Geometry: final body of the model. Coordinates: model frame, mm. Face numbers are marked on the shaded views. A direction names the side the tool comes from. Give positions to 0.01 mm unless a question says otherwise; leave off trailing zeros. Write each loop counter-clockwise with the first axis right and the second up, starting at its lowest first coordinate (ties: lowest second). Pieces come first, ordered by that corner, then holes.
from build123d import *

# Parameters (mm, degrees)
SKETCH5_R          = 25
CUT_EXTRUDE2_DEPTH = 100
SKETCH6_W          = 54.11225924
SKETCH6_H          = 36.891131312
CUT_EXTRUDE3_DEPTH = 75


with BuildPart() as part:
    # Sketch4 → Revolve2 (revolve)
    with BuildSketch(Plane.XY, mode=Mode.PRIVATE) as revolve2_sk:
        Polygon((0, -251.612903226), (0, -151.612903226), (100, -151.612903226), (100, 48.387096774), (152.822580645, 48.387096774), (200, 48.387096774), (200, -1.612903226), (150, -1.612903226), (150, -151.612903226), (300, -151.612903226), (300, -251.612903226), align=None)
    revolve(revolve2_sk.sketch.rotate(Axis((0, -251.612903226, 0), (0, 1, 0)), 90), axis=Axis((0, -251.612903226, 0), (0, 1, 0)))

    # Sketch5 → Cut-Extrude2 (cut)
    with BuildSketch(Plane(origin=(0, -151.612903226, 0), x_dir=(1, 0, 0), z_dir=(0, 1, 0))):
        with Locations(Location((0, 255.365455535, 0), (0, 0, 270))):
            Circle(SKETCH5_R)
        with Locations(Location((255.365455535, 0, 0), (0, 0, 270))):
            Circle(SKETCH5_R)
        with Locations(Location((0, -255.365455535, 0), (0, 0, 270))):
            Circle(SKETCH5_R)
        with Locations(Location((-255.365455535, 0, 0), (0, 0, 270))):
            Circle(SKETCH5_R)
    extrude(amount=-CUT_EXTRUDE2_DEPTH, mode=Mode.SUBTRACT)

    # Sketch6 → Cut-Extrude3 (cut)
    with BuildSketch(Plane(origin=(0, 48.387096774, 0), x_dir=(1, 0, 0), z_dir=(0, 1, 0))):
        with Locations((200, 0)):
            Rectangle(SKETCH6_W, SKETCH6_H)
    extrude(amount=-CUT_EXTRUDE3_DEPTH, mode=Mode.SUBTRACT)


solid = part.part
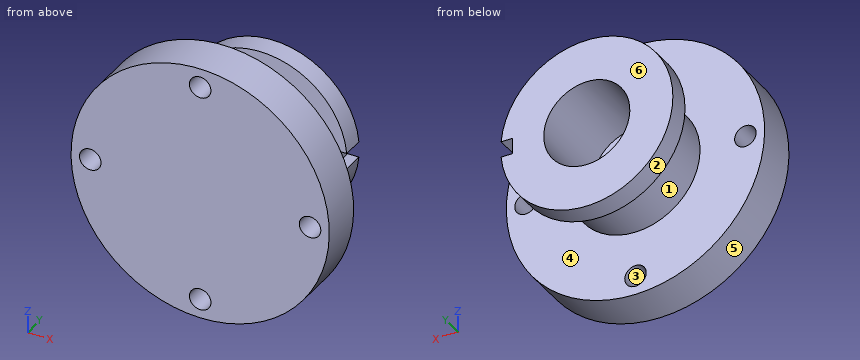
Q1. Section D-D on x = 263. Output: boundary loops of the cut face in (y, z).
Filled sheet:
outline: (-251.61, -144.33) - (-151.61, -144.33) - (-151.61, -23.81) - (-251.61, -23.81) - close; (-251.61, 23.81) - (-151.61, 23.81) - (-151.61, 144.33) - (-251.61, 144.33) - close
Q2. Section A-A on z = 0. Output: boundary loops of the cut face in (x, y), plus the area to 3 significant figures.
Filled sheet:
outline: (-300, -251.61) - (-280.37, -251.61) - (-280.37, -151.61) - (-300, -151.61) - close; (-230.37, -251.61) - (230.37, -251.61) - (230.37, -151.61) - (150, -151.61) - (150, -1.61) - (172.94, -1.61) - (172.94, 48.39) - (100, 48.39) - (100, -151.61) - (-100, -151.61) - (-100, 48.39) - (-200, 48.39) - (-200, -1.61) - (-150, -1.61) - (-150, -151.61) - (-230.37, -151.61) - close; (280.37, -251.61) - (300, -251.61) - (300, -151.61) - (280.37, -151.61) - close
area: 73,600 mm2
Q3. Ray query, line 1 along X through (y, z) = (-199, 0); line 2 along Y through (x, z) = (151, 13); line 3 along Z through (x, y) = (-3, -101). Return the intervals inside material, ascending.
Filled sheet:
line 1: x = -300 to -280.37, -230.37 to 230.37, 280.37 to 300
line 2: y = -251.61 to -151.61, -1.61 to 48.39
line 3: z = -149.97 to -99.95, 99.95 to 149.97
Q4. Section C-C on y = -42.5. Output: boundary loops of the cut face in (x, z).
Filled sheet:
outline: circle Ø300 at (0, 0); hole circle Ø200 at (0, 0)
Q5. Access query for the marked faces 1, 2 and 3. Directions: +Z, -Z, +X, -X, +Y, -Y. A direction counts if a zero-diameter tool reaches every point of the face in a straight line with its end or side. Return the directions, or none.
Filled sheet:
face 1: none
face 2: +Y
face 3: +Y, -Y
Q6. Section B-B on x = 0. Output: boundary loops of the cut face in (y, z).
Filled sheet:
outline: (-251.61, -300) - (-151.61, -300) - (-151.61, -280.37) - (-251.61, -280.37) - close; (-251.61, -230.37) - (-151.61, -230.37) - (-151.61, -150) - (-1.61, -150) - (-1.61, -200) - (48.39, -200) - (48.39, -100) - (-151.61, -100) - (-151.61, 100) - (48.39, 100) - (48.39, 200) - (-1.61, 200) - (-1.61, 150) - (-151.61, 150) - (-151.61, 230.37) - (-251.61, 230.37) - close; (-251.61, 280.37) - (-151.61, 280.37) - (-151.61, 300) - (-251.61, 300) - close
Q7. Pull-direction query (Y, two-part tool) for the marked faces 4, 5 and 6; classes: released by +Y, released by -Y, zero draft, split by the parting line, or undercut.
Filled sheet:
face 4: undercut
face 5: zero draft
face 6: released by +Y
Q8. Pin query (flat end, axial travel): P1, Ø8, axis at x = 183.5, y = 22.5, coming from the -Z side; P2, Ø11, axis at y = 16.5, z = 7.5, coming from the +X side; P3, Ø1, axis at y = -5.5, z = -113, coming from the +X side. Return the tip coordinate at first contact, or that it passes through.
Filled sheet:
P1: stops at z = -88.2
P2: stops at x = 172.94
P3: stops at x = 99.22
